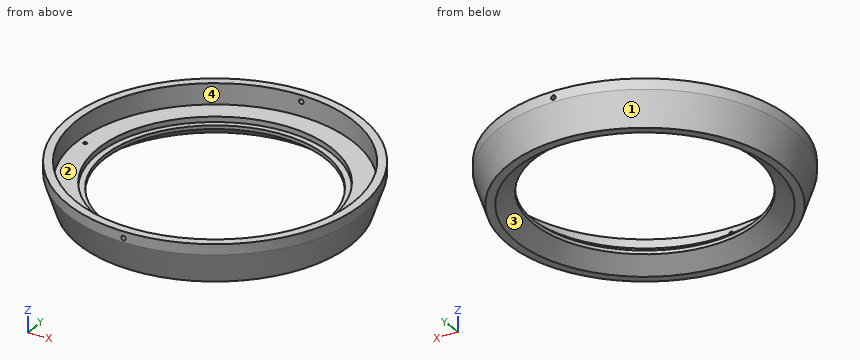
```python
from build123d import *

# Parameters (mm, degrees)
SKETCH1_R                     = 88.265
BOSS_EXTRUDE1_DEPTH           = 25.4
SKETCH2_R                     = 83.185
CUT_EXTRUDE1_DEPTH            = 9.144
SKETCH3_R                     = 76.2
CUT_EXTRUDE2_DEPTH            = 3.302
SKETCH4_R                     = 70.231
CUT_EXTRUDE3_DEPTH            = 3.175
SKETCH6_R                     = 66.675
CUT_EXTRUDE5_DEPTH            = 126.799189548
SKETCH7_R                     = 83.185
CUT_EXTRUDE6_DEPTH            = 3.302
CHAMFER2_SIZE                 = 6.35
CHAMFER2_SIZE2                = 19.05
CHAMFER1_SIZE                 = 7.62
CHAMFER1_SIZE2                = 10.16
CUT_EXTRUDE4_DEPTH            = 128.383595686
CUT_EXTRUDE4_DEPTH_BACK       = 128.383595686
SKETCH5_R                     = 1.35255
TAP_DRILL_FOR_4_40_TAP1_D     = 2.2606
TAP_DRILL_FOR_4_40_TAP1_DEPTH = 6.35
TAP_DRILL_FOR_4_40_TAP1_TIP   = 0.679152758


with BuildPart() as part:
    # Sketch1 → Boss-Extrude1 (new body)
    with BuildSketch(Plane.XY):
        Circle(SKETCH1_R)
    extrude(amount=BOSS_EXTRUDE1_DEPTH)

    # Sketch2 → Cut-Extrude1 (cut)
    with BuildSketch(Plane.XY.offset(25.4)):
        Circle(SKETCH2_R)
    extrude(amount=-CUT_EXTRUDE1_DEPTH, mode=Mode.SUBTRACT)

    # Sketch3 → Cut-Extrude2 (cut)
    with BuildSketch(Plane.XY.offset(16.256)):
        Circle(SKETCH3_R)
    extrude(amount=-CUT_EXTRUDE2_DEPTH, mode=Mode.SUBTRACT)

    # Sketch4 → Cut-Extrude3 (cut)
    with BuildSketch(Plane.XY.offset(12.954)):
        Circle(SKETCH4_R)
    extrude(amount=-CUT_EXTRUDE3_DEPTH, mode=Mode.SUBTRACT)

    # Sketch6 → Cut-Extrude5 (cut, through all)
    with BuildSketch(Plane.XY.offset(9.779)):
        Circle(SKETCH6_R)
    extrude(amount=-CUT_EXTRUDE5_DEPTH, mode=Mode.SUBTRACT)

    # Sketch7 → Cut-Extrude6 (cut)
    with BuildSketch(Plane.XY.offset(16.256)):
        Circle(SKETCH7_R)
    extrude(amount=-CUT_EXTRUDE6_DEPTH, mode=Mode.SUBTRACT)

    # Chamfer2
    chamfer2_edges = [part.edges().sort_by_distance(p)[0] for p in [
        (-88.265, 0, 0),
    ]]
    chamfer2_side = [part.faces().sort_by_distance(p)[0] for p in [
        (-85.768488798, 0, 0),
    ]]
    chamfer(chamfer2_edges, length=CHAMFER2_SIZE, length2=CHAMFER2_SIZE2, reference=chamfer2_side[0])

    # Chamfer1
    chamfer1_edges = [part.edges().sort_by_distance(p)[0] for p in [
        (-66.675, 0, 0),
    ]]
    chamfer1_side = [part.faces().sort_by_distance(p)[0] for p in [
        (-66.675, 0, 4.8895),
    ]]
    chamfer(chamfer1_edges, length=CHAMFER1_SIZE, length2=CHAMFER1_SIZE2, reference=chamfer1_side[0])

    # Sketch5 → Cut-Extrude4 (cut, two sides: drawn at the far end of the back side and taken through both)
    with BuildSketch(Plane(origin=(0, 0, 0), x_dir=(1, 0, 0), z_dir=(0, 1, 0)).offset(-CUT_EXTRUDE4_DEPTH_BACK)):
        with Locations(Location((0, -21.59, 0), (0, 0, 270))):
            Circle(SKETCH5_R)
    extrude(amount=CUT_EXTRUDE4_DEPTH + CUT_EXTRUDE4_DEPTH_BACK, mode=Mode.SUBTRACT)

    # Tap Drill for #4-40 Tap1
    with Locations(Plane.XY.offset(12.954)):
        with Locations((-78.74, 0), (78.74, 0)):
            Hole(TAP_DRILL_FOR_4_40_TAP1_D / 2, depth=TAP_DRILL_FOR_4_40_TAP1_DEPTH)
            with Locations((0, 0, -(TAP_DRILL_FOR_4_40_TAP1_DEPTH + TAP_DRILL_FOR_4_40_TAP1_TIP / 2))):  # 118° drill point
                Cone(0, TAP_DRILL_FOR_4_40_TAP1_D / 2, TAP_DRILL_FOR_4_40_TAP1_TIP, mode=Mode.SUBTRACT)


solid = part.part
```
Geometry: final body of the model. Coordinates: model frame, mm. Face numbers are marked on the shaded views. A direction names the side the tool comes from. Give positions to 0.01 mm unless a question says otherwise; leave off trailing zeros. Loops run counter-clockwise (first coordinate to the right, second up) from the corner with the lowest first, then second, coordinate; pieces in that order, holes last. Notation, with made-up numbers: (15.5, 35.5) - (67.5, 35.5) arc R13 ccw to (67.5, 55.5) - close; hole circle Ø10 at (60.25, -34.75). An arc over 180 degrees is marked (long way). Answer as CSV lines item,"result". Start each with the question number.
(1) Pin query (flat end, axial travel): P1, Ø4, axis at y = 56, z = 6, coming from the -X side; P2, Ø8, axis at y = -34.5, z = 13, coming from the -X side; P3, Ø2, axis at y = -38.5, z = 4.5, coming from the +X side; P4, Ø1.8, axis at x = -78.74, y = 0, coming from the -Z side. Return the tip coordinate at first contact, or that it passes through.
(2) Ray query, line 1 along Y through (x, z) = (47.5, 10); line 2 along Y through (x, z) = (-56, 14.75); line 3 along X through (y, z) = (-62.5, 18.25). Return the intervals inside material, ascending. Write a range as [from, to].
(3) Section query A-A (z = 2.75). Output: boundary loops of the cut face in (x, y), and give its area (3 significant figures).
(4) Section query B-B (z = 16.5). Output: boundary loops of the cut face in (x, y) (3 decimals).
(5) Mould query, pull axis X, two halves, no side actions, for the marked faces 1 and 2. Classes: +X half, -X half, draft (parallel to the pull), parting line (faces both ways), or undercut.
(6) Reachability of the marked faces 3 and 4 from +Z, -Z, +X, -X, +Y, -Y: full face, straight path, thin tool, end or side. Return the list, or none.
Worked answers:
1,P1,"stops at x = -64.44"
1,P2,"stops at x = -81.24"
1,P3,"stops at x = 74.63"
1,P4,"stops at z = 0"
2,line 1,"y = [-70.79, -51.73], [51.73, 70.79]"
2,line 2,"y = [-66.36, -61.51], [61.51, 66.36]"
2,line 3,"x = [-61.95, -54.9], [54.9, 61.95]"
3,outline,"circle Ø165.66 at (0, 0); hole circle Ø146.34 at (0, 0)"
3,area,"4,740 mm^2"
4,outline,"circle Ø174.83 at (0, 0); hole circle Ø166.37 at (0, 0)"
5,face 1,"parting line"
5,face 2,"undercut"
6,face 3,"-Z"
6,face 4,"+Z"
